Source: CAD feature listing. Evaluate the final solid. Frame: model axes, mm. A direction names the side the tool comes from. Give positions to 0.01 mm unless a question says otherwise; leave off trailing zeros. Put each result on its own line as item: value.
```python
from build123d import *

# Parameters (mm, degrees)
F0_R     = 5
F0_R_2   = 3
F1_DEPTH = 0.4
F3_R     = 3.05
F3_R_2   = 1.525
F6_SIZE  = 0.2
F7_R     = 0.4


# Not quite as in the source:
# - a fillet or chamfer that OpenCascade refuses, or shapes differently, is made with other operations: its cross-section is extruded or revolved along the edge and cut away or added


with BuildPart() as f1:
    # F0 (on Top) → F1 (new body)
    with BuildSketch(Plane.XY):
        Circle(F0_R)
        Circle(F0_R_2, mode=Mode.SUBTRACT)
    extrude(amount=F1_DEPTH)

    # F4: sweep along a path in F2
    with BuildLine(Plane.YZ) as f4_path:
        Line((0, 0), (0, 4))
        ThreePointArc((0, 4), (-0.1090373559, 4.8282209443), (-0.4287187079, 5.6))
        Line((-0.4287187079, 5.6), (-2.9287187079, 9.9301270189))
    # F3 (on Top) → F4 (sweep)
    with BuildSketch(Plane.XY):
        Circle(F3_R)
        Circle(F3_R_2, mode=Mode.SUBTRACT)
    sweep(path=f4_path.line)

    # F5: fillet of radius 3 on 1 edges, made by hand

    # F5_s1 → F5_t2 (revolve)
    with BuildSketch(Plane.XZ):
        with BuildLine():
            ThreePointArc((5, 0.4), (3.5852484912, 1.4999859616), (3.05, 3.2102490993))
            Line((3.05, 3.2102490993), (3.05, 0.4))
            Line((3.05, 0.4), (5, 0.4))
        make_face()
    revolve(axis=Axis((0, 0, 0.4), (0, 0, 1)))

    # F6
    f6_edges = [f1.edges().sort_by_distance(p)[0] for p in [
        (-5, 0, 0),
        (-1.525, 0, 0),
    ]]
    chamfer(f6_edges, length=F6_SIZE)

    # F7
    f7_edges = [f1.edges().sort_by_distance(p)[0] for p in [
        (-3.05, -2.928719, 9.930127),
    ]]
    fillet(f7_edges, radius=F7_R)


solid = f1.part
```
(1) Draft query along Y for faces 3 (the cylindrical face through (-0.397, 1.024, 9.132)), 4 (the flat face through (2, 0, 0)), 5 (the cylindrical face through (-1.524, 0.067, 2.127)), 6 (the cylindrical face through (0, -3, 7)). Return one class per face: released by +Y, released by -Y, zero draft, split by the parting line, or undercut.
Calculated:
face 3: split by the parting line
face 4: zero draft
face 5: undercut
face 6: undercut
(2) Line query: probe 1 along Y at (x, z) = (0, 2.35) (3 decimals); probe 2 along Z at (x, y) = (-0.75, -4.5); probe 3 along X at (y, z) = (0.5, 3). Output: solid intervals per line, ascending. Write a range as from..to.
Calculated:
probe 1: y = -3.176..-1.525, 1.525..3.176
probe 2: z = 0..0.61, 6.74..9.02
probe 3: x = -3.02..-1.44, 1.44..3.02
(3) First-contact query: P1, Ø1.5, axis at y = 3, z = 1.5, coming from the +X side; P2, Ø3, axis at y = 2.5, z = 8, coming from the +X side; P3, Ø6, axis at x = -1.5, z = 10, coming from the +Y side. Flat tips, straight axial feed; report the tip coordinate or a pass-through.
Calculated:
P1: stops at x = 3.28
P2: stops at x = 2.07
P3: stops at y = 2.14
(4) Reachability of faces 1 (the flat face through (-0.037, -1.431, 10.795)), 2 (the cylindrical face through (-3.047, 0.134, 3.611)) from +Z, -Z, +X, -X, +Y, -Y: full face, straight path, thin tool, end or side. Return the list, or none.
Calculated:
face 1: +Z, +X, -X, -Y
face 2: none
